Verification items for the finished model (mm, model axes). A direction names the side the tool comes from. Coordinates: 2 decimals unless noted, no trailing zeros. Order: outer loops, then holes, each group sorted by start corner. A loop starts at its lowest first (then second) coordinate and runs counter-clockwise, first axis right, second up.
Q1. Depth check by flat-ended pin: P1, Ø4.5, axis at x = 69, z = 9.5, coming from the -Y side; P2, Ø5, axis at x = 18.5, z = 27.5, coming from the +Y side; P3, Ø8, axis at y = 27.5, z = 13.5, coming from the +X side. Enter the tip coordinate at first touch or a pass-through.
Q2. Cross-section at A-A, the plane y = -24.5. Record the boundary of the cut face in (x, z).
Q3. Thickness scan on line 1 (X direction, y = -53.5, z = 12); line 2 (Y direction, x = 45, z = 17). Record the ranges inside material, lowest first.
Q4. Draft check along Y on faces 5 (the cylindrical face through (-59.14, -59.1, 19.73)), 6 (the flat face through (61, 28.1, 1.3)), 7 (the flat face through (1, 1, 39)). Enter one of: pulls with the +Y half, pulls with the -Y half, needs draft (parallel to the pull), parting line crosses it, or undercut.
Q5. Set-up check for faces 1 (the cylindrical face through (75.055, -0.014, 7.877)), 2 (the cylindrical face through (-59.1, 59.14, 19.73)), 3 (the flat face through (62, -30, 1)), 4 (the flat face through (61, -31.9, 1.3)): record each of +Z, -Z, +X, -X, +Y, -Y from which the full face is reachable in a straight line by a thin tool's end or side.
Q6. Cross-section at B-B, the plane z = 29. Record the boundary of the cut face in (x, y), and give its area (3 significant figures).
from build123d import *

# Parameters (mm, degrees)
PAD_DEPTH       = 39
PAD001_DEPTH    = 1
SKETCH002_W     = 51
SKETCH002_H     = 16
PAD002_DEPTH    = 2
SKETCH003_W     = 46
SKETCH003_H     = 14
POCKET_DEPTH    = 3
SKETCH004_W     = 49
SKETCH004_H     = 15
POCKET001_DEPTH = 1
PAD003_DEPTH    = 1


with BuildPart() as part:
    # Sketch → Pad (new body)
    with BuildSketch(Plane.XY):
        with BuildLine():
            Line((-57, 60), (57, 60))
            ThreePointArc((60, 57), (59.12132, 59.12132), (57, 60))
            Line((60, 57), (60, -57))
            ThreePointArc((57, -60), (59.12132, -59.12132), (60, -57))
            Line((57, -60), (-57, -60))
            ThreePointArc((-60, -57), (-59.12132, -59.12132), (-57, -60))
            Line((-60, -57), (-60, 57))
            ThreePointArc((-57, 60), (-59.12132, 59.12132), (-60, 57))
        make_face()
    extrude(amount=PAD_DEPTH)

    # Sketch001 → Pad001 (join)
    with BuildSketch(Plane.XY):
        with BuildLine():
            Line((-60, 63), (47, 63))
            ThreePointArc((50, 60), (49.12132, 62.12132), (47, 63))
            Line((50, 60), (50, -60))
            ThreePointArc((47, -63), (49.12132, -62.12132), (50, -60))
            Line((47, -63), (-60, -63))
            Line((-60, -63), (-60, 63))
        make_face()
    extrude(amount=PAD001_DEPTH)

    # Sketch002 (on Face19 of Pad001) → Pad002 (join)
    with BuildSketch(Plane.YZ.offset(60)):
        with Locations((-30, 8)):
            Rectangle(SKETCH002_W, SKETCH002_H)
        with Locations((30, 8)):
            Rectangle(SKETCH002_W, SKETCH002_H)
    extrude(amount=PAD002_DEPTH)

    # Sketch003 (on DatumPlane) → Pocket (cut)
    with BuildSketch(Plane.YZ.offset(60)):
        with Locations((-30, 9)):
            Rectangle(SKETCH003_W, SKETCH003_H)
        with Locations((30, 9)):
            Rectangle(SKETCH003_W, SKETCH003_H)
    extrude(amount=POCKET_DEPTH, mode=Mode.SUBTRACT)

    # Sketch004 (on DatumPlane) → Pocket001 (cut)
    with BuildSketch(Plane.YZ.offset(60)):
        with Locations((-30, 8.5)):
            Rectangle(SKETCH004_W, SKETCH004_H)
        with Locations((30, 8.5)):
            Rectangle(SKETCH004_W, SKETCH004_H)
    extrude(amount=POCKET001_DEPTH, mode=Mode.SUBTRACT)

    # Sketch005 → Pad003 (join, symmetric)
    with BuildSketch(Plane.XZ):
        with BuildLine():
            ThreePointArc((72, 0), (75.055728, 8), (72, 16))
            Line((72, 16), (60, 16))
            Line((60, 16), (60, 0))
            Line((60, 0), (72, 0))
        make_face()
    extrude(amount=PAD003_DEPTH, both=True)


solid = part.part
Check values:
1. P1: stops at y = -1
1. P2: stops at y = 60
1. P3: stops at x = 60
2. outline: (-60, 0) - (62, 0) - (62, 2) - (61, 2) - (61, 1) - (60, 1) - (60, 39) - (-60, 39) - close
3. line 1: x = -60 to 60, 61 to 62
3. line 2: y = -60 to 60
4. face 5: pulls with the -Y half
4. face 6: undercut
4. face 7: needs draft
5. face 1: +X, +Y, -Y
5. face 2: +Z, -X, +Y
5. face 3: +Z, -Z, +X, -Y
5. face 4: +Z
6. outline: (-60, -57) arc R3 ccw to (-57, -60) - (57, -60) arc R3 ccw to (60, -57) - (60, 57) arc R3 ccw to (57, 60) - (-57, 60) arc R3 ccw to (-60, 57) - close
6. area: 14,400 mm2
